Read the model definition and answer for the solid it produces. Units are mm, in the model's axes. A direction names the side the tool comes from. Give positions to 0.01 mm unless a question says otherwise; leave off trailing zeros. Write each loop counter-clockwise with the first axis right and the second up, starting at its lowest first coordinate (ties: lowest second). Pieces come first, ordered by that corner, then holes. Notation, with made-up numbers: (-11, 8) -> (39, 8) arc R12 ccw to (39, 19) -> close; hole circle Ø1 at (42, 9.5). An arc over 180 degrees is marked (long way). Write item = value, one per line.
from build123d import *

# Parameters (mm, degrees)
F0_W         = 141.1362439394
F0_H         = 15.875
F1_DEPTH     = 25.4
F2_SIZE      = 1.27
F3_T         = 3.81
F3_T3_DEPTH  = 31.75
F3_T5_DEPTH  = 10.3365589148
F3_T7_DEPTH  = 33.02
F3_T9_DEPTH  = 9.8197045256
F3_T11_DEPTH = 9.8197045256
F4_R         = 4.1275
F4_R_2       = 1.8415
F5_DEPTH     = 21.59


# Not quite as in the source:
# - a shell that OpenCascade refuses in one call is made with other operations: the cavity is built on its own and cut out
# - a feature names something its author has since deleted; it is built from what else it names


with BuildPart() as f1:
    # F0 (on Front) → F1 (new body)
    with BuildSketch(Plane.XZ):
        Polygon((115.6852519128, 43.8017650865), (-71.6397480872, 43.8017650865), (-71.6397480872, -48.2732349135), (-30.3647480872, -48.2732349135), (-30.3647480872, -28.973974956), (109.3352519128, -28.973974956), (109.3352519128, -48.2732349135), (150.6102519128, -48.2732349135), (150.6102519128, -22.8732349135), (132.2698407767, -12.0163811026), (150.6102519128, 0), (150.6102519128, 28.575), align=None)
        with Locations((37.9095822573, 10.4642650865)):
            Rectangle(F0_W, F0_H, mode=Mode.SUBTRACT)
    extrude(amount=F1_DEPTH)

    # F2
    f2_edges = [f1.edges().sort_by_distance(p)[0] for p in [
        (-71.639748, -25.4, -2.235735),
        (22.022752, -25.4, 43.801765),
        (133.147752, -25.4, 36.188383),
        (150.610252, -25.4, 14.2875),
        (141.440046, -25.4, -6.008191),
        (141.440046, -25.4, -17.444808),
        (150.610252, -25.4, -35.573235),
        (129.972752, -25.4, -48.273235),
        (109.335252, -25.4, -38.623605),
        (39.485252, -25.4, -28.973975),
        (-30.364748, -25.4, -38.623605),
        (-51.002248, -25.4, -48.273235),
    ]]
    chamfer(f2_edges, length=F2_SIZE)

    # F3: shell of thickness 3.81, made by hand


with BuildPart() as f3_core1:
    # F3_t2: copy of F1
    add(f1.part)

    # the walls: a layer under each face that stays
    f3_faces = [f3_core1.faces().sort_by_distance(p)[0] for p in [
        (141.4400463447, -12.065, -17.4448080081),
        (150.6102519128, -12.065, -35.5732349135),
        (140.2396500387, -24.765, -17.4721355193),
        (141.4400463447, -12.065, -6.0081905513),
        (129.9727519128, -12.065, -48.2732349135),
        (149.9752519128, -24.765, -35.5732349135),
        (39.4852519128, -25.4, -2.2357349135),
        (140.2396500387, -24.765, -6.0355180626),
        (150.6102519128, -12.065, 14.2875),
        (133.1477519128, -12.065, 36.1883825433),
        (22.0227519128, -12.065, 43.8017650865),
        (-71.6397480872, -12.065, -2.2357349135),
        (-51.0022480872, -12.065, -48.2732349135),
        (-30.3647480872, -12.065, -38.6236049347),
        (39.4852519128, -12.065, -28.973974956),
        (109.3352519128, -12.065, -38.6236049347),
        (-32.6585397124, -12.7, 10.4642650865),
        (37.9095822573, -12.7, 18.4017650865),
        (108.477704227, -12.7, 10.4642650865),
        (37.9095822573, -12.7, 2.5267650865),
        (129.9727519128, -24.765, -47.6382349135),
        (-71.0047480872, -24.765, -2.2357349135),
        (22.0227519128, -24.765, 43.1667650865),
        (-51.0022480872, -24.765, -47.6382349135),
        (132.8939724947, -24.765, 35.6062992099),
        (-30.9997480872, -24.765, -37.9886049347),
        (149.9752519128, -24.765, 14.2875),
        (39.4852519128, -24.765, -28.338974956),
        (109.9702519128, -24.765, -37.9886049347),
    ]]
    thicken(f3_faces, amount=-F3_T, mode=Mode.SUBTRACT)

    # F3_s4 → F3_t3 (cut)
    with BuildSketch(Plane.XZ.offset(-3.81)):
        Polygon((132.3101290844, -12.0154639229), (130.3290203992, -15.2949960941), (125.0674629404, -12.1803461703), (130.1818303825, -8.8294840861), align=None)
        Polygon((-30.3266480872, -29.012074956), (-34.1747480872, -28.973974956), (-34.1747480872, -25.163974956), (-30.3647480872, -25.163974956), align=None)
        Polygon((109.2971519128, -29.012074956), (109.3352519128, -25.163974956), (113.1452519128, -25.163974956), (113.1452519128, -28.973974956), align=None)
    extrude(amount=F3_T3_DEPTH, mode=Mode.SUBTRACT)

    # F3_s6 → F3_t5 (cut)
    with BuildSketch(Plane(origin=(96.491386595, 51.0431681427, 2.1966657526), x_dir=(0.4675978526, -0.8839413149, 0), z_dir=(-0.8837623948, -0.4675032053, -0.0201192112))):
        Polygon((83.2395465479, -14.1386059374), (80.1554756401, -16.4580548587), (78.415785798, -14.1899447458), (80.1068084957, -11.8853218988), align=None)
    extrude(amount=F3_T5_DEPTH, mode=Mode.SUBTRACT)

    # F3_s8 → F3_t7 (cut)
    with BuildSketch(Plane.XZ.offset(-3.81)):
        Polygon((-32.6204397124, 2.5648650865), (-36.4685397124, 2.5267650865), (-36.4685397124, -1.2832349135), (-32.6585397124, -1.2832349135), align=None)
        Polygon((-32.6204397124, 18.3636650865), (-36.4685397124, 18.4017650865), (-36.4685397124, 22.2117650865), (-32.6585397124, 22.2117650865), align=None)
        Polygon((108.439604227, 18.3636650865), (108.477704227, 22.2117650865), (112.287704227, 22.2117650865), (112.287704227, 18.4017650865), align=None)
        Polygon((108.439604227, 2.5648650865), (112.287704227, 2.5267650865), (112.287704227, -1.2832349135), (108.477704227, -1.2832349135), align=None)
    extrude(amount=F3_T7_DEPTH, mode=Mode.SUBTRACT)

    # F3_s10 → F3_t9 (cut)
    with BuildSketch(Plane(origin=(-6.3072198515, -6.3072198515, 6.3072198515), x_dir=(0.7071067812, -0.7071067812, 0), z_dir=(-0.5773502692, -0.5773502692, 0.5773502692))):
        Polygon((-4.3514826515, -45.9375348012), (-8.2186326515, -45.9045392333), (-8.2186326515, -43.7048347077), (-6.3136326515, -42.6049824449), align=None)
    extrude(amount=F3_T9_DEPTH, mode=Mode.SUBTRACT)

    # F3_s12 → F3_t11 (cut)
    with BuildSketch(Plane(origin=(32.6307211267, -32.6307211267, 32.6307211267), x_dir=(0.7071067812, 0.7071067812, 0), z_dir=(0.5773502692, -0.5773502692, 0.5773502692))):
        Polygon((60.1920614202, -78.177107985), (62.1542114202, -74.8445556287), (64.0592114202, -75.9444078915), (64.0592114202, -78.1441124172), align=None)
    extrude(amount=F3_T11_DEPTH, mode=Mode.SUBTRACT)


with BuildPart() as f1_1:
    add(f1.part)

    # what is left inside the walls is the cavity
    f3_cavity = [f3_core1.part.solids().sort_by_distance(p)[0] for p in [
        (39.485252, -21.5519, -16.311568),
    ]]
    add(f3_cavity, mode=Mode.SUBTRACT)

    # F4 (on face) → F5 (join, through all)
    with BuildSketch(Plane(origin=(0, -21.59, 0), x_dir=(-1, 0, 0), z_dir=(0, 1, 0))):
        with Locations((48.7797480872, 21.8307650865)):
            Circle(F4_R)
        with Locations((48.7797480872, 21.8307650865)):
            Circle(F4_R_2, mode=Mode.SUBTRACT)
        with Locations((48.7797480872, -28.8422349135)):
            Circle(F4_R)
        with Locations((48.7797480872, -28.8422349135)):
            Circle(F4_R_2, mode=Mode.SUBTRACT)
        with Locations((-125.7182519128, 19.8926216617)):
            Circle(F4_R)
        with Locations((-125.7182519128, 19.8926216617)):
            Circle(F4_R_2, mode=Mode.SUBTRACT)
        with Locations((-125.7182519128, -31.1790349135)):
            Circle(F4_R)
        with Locations((-125.7182519128, -31.1790349135)):
            Circle(F4_R_2, mode=Mode.SUBTRACT)
    extrude(amount=F5_DEPTH)


solid = f1_1.part
(1) Consider L1, parallel to Z at x = 59, y = -11.25; L2, parallel to X at y = -17.5, z = 8; L3, parallel to X at y = -20.5, z = 0. Determine where each line is inside the solid, lowest interval first.
Checks:
L1 = -28.97 to -25.16, -1.28 to 2.53, 18.4 to 22.21, 39.99 to 43.8
L2 = -71.64 to -67.83, -36.47 to -32.66, 108.48 to 112.29, 146.8 to 150.61
L3 = -71.64 to -67.83, -36.47 to 112.29, 143.66 to 150.61
(2) The part is cut by section A-A on z = 6.5. Determine the outline of the cut face in (x, y).
Checks:
outline = (-71.64, -24.13) -> (-70.37, -25.4) -> (-32.66, -25.4) -> (-32.66, 0) -> (-36.47, 0) -> (-36.47, -21.59) -> (-67.83, -21.59) -> (-67.83, 0) -> (-71.64, 0) -> close; (108.48, -25.4) -> (149.34, -25.4) -> (150.61, -24.13) -> (150.61, 0) -> (146.8, 0) -> (146.8, -21.59) -> (112.29, -21.59) -> (112.29, 0) -> (108.48, 0) -> close
(3) For a pull along X with two mould halves and no side action, classify faces 5 (the flat face through (141.57, -11.9, -17.52)), 6 (the flat face through (-51, -11, -44.463)), 7 (the flat face through (130, -11, -44.463)), 8 (the flat face through (130, -12, -48.273)) as released by +X, released by -X, zero draft, split by the parting line, or undercut.
Checks:
face_5 = released by +X
face_6 = undercut
face_7 = undercut
face_8 = zero draft
(4) The part is cut by section C-C on y = -6.75. Count the separate pieces of the cut face and the enclosed holes in it, plus the area to 3 significant figures.
Checks:
separate_pieces = 6
enclosed_holes = 6
area = 3,950 mm²
(5) The part is cut by section B-B on x = 47.5. Determine the outline of the cut face in (y, z).
Checks:
outline = (-25.4, -27.7) -> (-24.13, -28.97) -> (0, -28.97) -> (0, -25.16) -> (-21.59, -25.16) -> (-21.59, -1.28) -> (0, -1.28) -> (0, 2.53) -> (-25.4, 2.53) -> close; (-25.4, 18.4) -> (0, 18.4) -> (0, 22.21) -> (-21.59, 22.21) -> (-21.59, 39.99) -> (0, 39.99) -> (0, 43.8) -> (-24.13, 43.8) -> (-25.4, 42.53) -> close
(6) A tool of negligible diameter and unlimited length cuts with its end or side. For faces 1 (the flat face through (140.38, -24.77, -17.56)), 2 (the cylindrical face through (-46.94, -10.95, 21.91)), 3 (the flat face through (37, -13, 18.402)), 4 (the flat face through (39, -12, -28.974)), from which of +Z, -Z, +X, -X, +Y, -Y can it reach the whole face along a straight path? Write none if from no direction.
Checks:
face_1 = +X, -Y
face_2 = +Y
face_3 = +Y, -Y
face_4 = -Z, +Y, -Y
(7) Given P1, Ø1.1, axis at x = 126, z = 20, coming from the +Y side; P2, Ø5, axis at y = -13, z = 33.5, coming from the +X side; P3, Ø6, axis at x = 28.5, z = 15.5, coming from the +Y side; P4, Ø12, axis at x = 17, y = -13, coming from the -Z side, each flat-ended and moving along its own axis, determine where each tip first touches the part or whether it passes through.
Checks:
P1 = -21.59
P2 = 145.05
P3 = 0
P4 = -28.97
